Part model, mm, in its own coordinate system. Face numbers are marked on the shaded views. A direction names the side the tool comes from. Round coordinates to 2 decimals unless told otherwise and drop trailing zeros. Write each loop counter-clockwise with the first axis right and the second up, starting at its lowest first coordinate (ties: lowest second). Pieces come first, ordered by that corner, then holes. Notation, with made-up numbers: (67, -9.75) -> (79, -9.75) arc R29 cw to (79, 29.25) -> close; hole circle Ø2 at (75, -3). An arc over 180 degrees is marked (long way). Use CSV: the item, a comma, the result in double quotes. Start each with the question number.
(1) Saw through at D-D (y = 11.5). Give the cut face in (x, z), plus the area to 3 significant figures.
(2) Saw through at C-C (x = -15). Give the cut face in (y, z).
(3) Drop flat-ended pins along their axis: pin 1 (10 mm diameter, centred on y = 35, z = 7.5, fed in from +X); pin 2 (9.5 mm diameter, centred on y = 11, z = 23.5, fed in from -X); pin 3 (7.5 mm diameter, centred on x = -17.5, z = 9, fed in from -Y). Give the stop position or say it passes through.
(4) Saw through at B-B (y = 37.5). Give the cut face in (x, z), plus the area to 3 significant figures.
(5) Which spindle directions (+Z, -Z, +X, -X, +Y, -Y) get a long thin tool onto all of the face, cutting with end or side? Do the marked faces 1 and 2. Say none if no direction does.
(6) Probe line 1 (Y direction, x = 0.75, z = 0); line 2 (Z direction, x = 0.05, y = 10); line 3 (X direction, y = 27, z = -46). List the from-to ranges inside material, lowest first. Write a range as [from, to].
(7) Saw through at A-A (z = 0). Give the cut face in (x, y).
(8) Two-plate mould, pull along X, no slides. Class the marked faces 3, 4 and 5: released by +X, released by -X, zero draft, split by the parting line, or undercut.
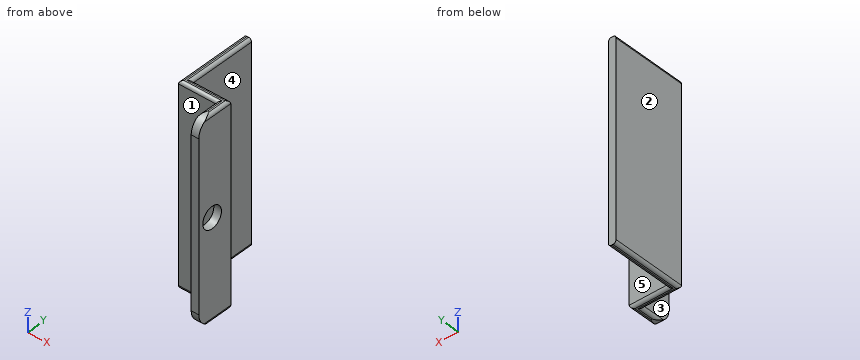
```python
from build123d import *

# Parameters (mm, degrees)
CUT_EXTRUDE1_DEPTH      = 99.145249503
CUT_EXTRUDE1_DEPTH_BACK = 99.145249503
SKETCH3_R               = 7
FILLET2_R               = 10
FILLET3_R               = 10


with BuildPart() as part:
    # Sweep1: sweep along a curve in space
    with BuildLine() as sweep1_path:
        Line((0, 0, 0), (0, 21.5, 0))
        Line((0, 21.5, 0), (-25, 21.5, 0))
        Line((-25, 21.5, 0), (-25, 68.2, 0))
    # Sketch2 → Sweep1 (sweep)
    with BuildSketch(Plane(origin=(0, 0, 0), x_dir=(1, 0, 0), z_dir=(0, 1, 0))):
        with BuildLine():
            Line((-0.5, 65), (0.5, 65))
            ThreePointArc((0.5, 65), (1.914213562, 64.414213562), (2.5, 63))
            Line((2.5, 63), (2.5, -63))
            ThreePointArc((2.5, -63), (1.914213562, -64.414213562), (0.5, -65))
            Line((0.5, -65), (-0.5, -65))
            ThreePointArc((-0.5, -65), (-1.914213562, -64.414213562), (-2.5, -63))
            Line((-2.5, -63), (-2.5, 63))
            ThreePointArc((-2.5, 63), (-1.914213562, 64.414213562), (-0.5, 65))
        make_face()
    sweep(path=sweep1_path.line, transition=Transition.RIGHT)

    # Sketch3 → Cut-Extrude1 (cut, two sides: drawn at the far end of the back side and taken through both)
    with BuildSketch(Plane(origin=(0, 0, 0), x_dir=(0, 0, -1), z_dir=(1, 0, 0)).offset(-CUT_EXTRUDE1_DEPTH_BACK)):
        with Locations((0, 10)):
            Circle(SKETCH3_R)
    extrude(amount=CUT_EXTRUDE1_DEPTH + CUT_EXTRUDE1_DEPTH_BACK, mode=Mode.SUBTRACT)

    # Fillet2
    # the kernel refuses this fillet: 10 mm, written as the material it takes off along each edge
    with BuildSketch(Plane(origin=(25.5, 0, -65), x_dir=(0, 1, 0), z_dir=(-1, 0, 0))) as fillet2_piece_1:
        with BuildLine():
            CenterArc((FILLET2_R, -FILLET2_R), FILLET2_R, 90, 90)
            Line((0, -FILLET2_R), (0, 0))
            Line((0, 0), (FILLET2_R, 0))
        make_face()
    extrude(amount=51, mode=Mode.SUBTRACT)

    # Fillet3
    # the kernel refuses this fillet: 10 mm, written as the material it takes off along each edge
    with BuildSketch(Plane(origin=(-25.5, 0, 65), x_dir=(0, 1, 0), z_dir=(1, 0, 0))) as fillet3_piece_1:
        with BuildLine():
            CenterArc((FILLET3_R, -FILLET3_R), FILLET3_R, 90, 90)
            Line((0, -FILLET3_R), (0, 0))
            Line((0, 0), (FILLET3_R, 0))
        make_face()
    extrude(amount=51, mode=Mode.SUBTRACT)


solid = part.part
```
Answers:
1,outline,"(-2.5, -63) arc R2 ccw to (-0.5, -65) -> (0.5, -65) arc R2 ccw to (2.5, -63) -> (2.5, -6.84) -> (-2.5, -6.84) -> close; (-2.5, 6.84) -> (2.5, 6.84) -> (2.5, 63) arc R2 ccw to (0.5, 65) -> (-0.5, 65) arc R2 ccw to (-2.5, 63) -> close"
1,area,"578 mm²"
2,outline,"(19, -63) arc R2 ccw to (21, -65) -> (22, -65) arc R2 ccw to (24, -63) -> (24, 63) arc R2 ccw to (22, 65) -> (21, 65) arc R2 ccw to (19, 63) -> close"
3,pin 1,"stops at x = -22.5"
3,pin 2,"stops at x = -2.5"
3,pin 3,"stops at y = 19"
4,outline,"(-27.5, -63) arc R2 ccw to (-25.5, -65) -> (-24.5, -65) arc R2 ccw to (-22.5, -63) -> (-22.5, 63) arc R2 ccw to (-24.5, 65) -> (-25.5, 65) arc R2 ccw to (-27.5, 63) -> close"
4,area,"647 mm²"
5,face 1,"+Z, -Z, -X, -Y"
5,face 2,"+Z, -Z, -X, +Y, -Y"
6,line 1,"y = [0, 3], [17, 24]"
6,line 2,"z = [-65, -7], [7, 65]"
6,line 3,"x = [-27.5, -22.5]"
7,outline,"(-27.5, 19) -> (-2.5, 19) -> (-2.5, 17) -> (2.5, 17) -> (2.5, 24) -> (-22.5, 24) -> (-22.5, 68.2) -> (-27.5, 68.2) -> close; (-2.5, 0) -> (2.5, 0) -> (2.5, 3) -> (-2.5, 3) -> close"
8,face 3,"released by -X"
8,face 4,"released by +X"
8,face 5,"zero draft"
